Here's how the part is built. I have some questions about the finished solid (model axes, mm). Round coordinates to 2 decimals unless told otherwise and drop trailing zeros. Write each loop counter-clockwise with the first axis right and the second up, starting at its lowest first coordinate (ties: lowest second). Pieces come first, ordered by that corner, then holes. Notation, with made-up numbers: M 23.25,-3.75 L 60.25,-3.75 A16 ccw 60.25,15.25 Z; hole C 17,-34.75 d4. An arc over 180 degrees is marked long. Use one line per item in the form item = value. Start each with the question number.
Q1. We'd pull the mould along Y, two halves only. Please class faces 1 (the face through (-1.17, -5.27, 1.77)), 2 (the face through (6.5, -2, 1.7)): +Y half, -Y half, draft (parallel to the pull), parting line (faces both ways), or undercut.
Q2. I need wall thicknesses on line 1 along Y through (x, z) = (0, 1.85); line 2 along Y through (x, z) = (0, 2.7); line 3 along X through (y, z) = (-4, 1.15). Which ranges of each line are inside material? Lowest first, please. Write a range as from..to.
Q3. I want a section at A-A on z = 1.85. List the corners of the cut face in (x, y) for me.
Q4. I want a section at B-B on z = 0.5. List the corners of the cut face in (x, y) for me.
Autodesk Fusion 360 part; units mm, degrees
sketch "スケッチ1" plane through (0, 0, 0) normal (0, 1, 0) x (1, 0, 0)
  line L0 (0, 0) -> (5.4, 0)
  line L1 (5.4, 0) -> (5.4, -3.5)
  line L2 (5.4, -3.5) -> (6.55, -3.5)
  line L3 (6.55, -3.5) -> (6.8, -2.25)
  line L4 (6.8, -2.25) -> (6.8, -1.25)
  line L5 (6.8, -1.25) -> (6.55, 0)
  line L6 (6.55, 0) -> (5.4, 0)
  dimension "d1" = 3.5
  dimension "d3" = 5.4
  dimension "d4" = 1
  dimension "d5" = 0.25
  dimension "d8" = 6.8
revolve "回転1" add sketch "スケッチ1" angle 360 about axis through (0, 0, 1.75) along (0, 0, 1)
fillet "フィレット1" radius 1 4 edges at (-6.1067, -2.3686, 0) (-6.3398, -2.459, 1.25) (-6.3398, -2.459, 2.25) (-6.1067, -2.3686, 3.5)
equation "d8 = ( 13.6 / 2 ) * 1 mm"
Reported:
q1.face_1 = undercut
q1.face_2 = parting line
q2.line_1 = -6.8..-5.4, 5.4..6.8
q2.line_2 = -6.71..-5.4, 5.4..6.71
q2.line_3 = -5.47..-3.63, 3.63..5.47
q3.outline = C 0,0 d13.6; hole C 0,0 d10.8
q4.outline = C 0,0 d13.19; hole C 0,0 d10.8
